Can you work these out from the model? Positions are in its coordinate system, mm. Round coordinates to 2 decimals unless told otherwise and drop trailing zeros. Loops run counter-clockwise (first coordinate to the right, second up) from the corner with the lowest first, then second, coordinate; pieces in that order, holes last. Notation, with made-up numbers: (-29, 72) -> (-7, 72) arc R21 ccw to (-7, 84) -> close; hole circle Ø9 at (-8.5, 80). An arc over 180 degrees is marked (long way). Answer as a JSON object with one key per item and string values.
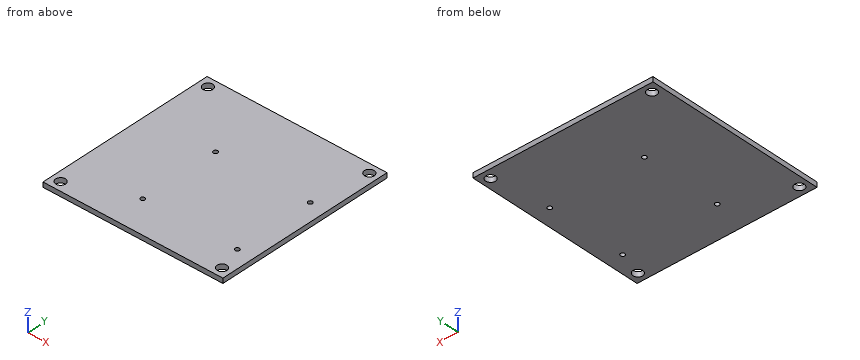
```python
from build123d import *

# Parameters (mm, degrees)
CROQUIS1_W              = 110.308657865
CROQUIS1_H              = 110.308657865
CROQUIS1_R              = 3
SALIENTE_EXTRUIR1_DEPTH = 3
CROQUIS3_R              = 1.35
CORTAR_EXTRUIR1_DEPTH   = 4


with BuildPart() as part:
    # Croquis1 → Saliente-Extruir1 (new body)
    with BuildSketch(Plane.XY.offset(1001.5)):
        with Locations((-24.891577249, 6.700344828)):
            Rectangle(CROQUIS1_W, CROQUIS1_H)
        with Locations((-74.389051931, 56.197819511)):
            Circle(CROQUIS1_R, mode=Mode.SUBTRACT)
        with Locations((24.605897435, -42.797129855)):
            Circle(CROQUIS1_R, mode=Mode.SUBTRACT)
        with Locations((-74.389051931, -42.797129855)):
            Circle(CROQUIS1_R, mode=Mode.SUBTRACT)
        with Locations((24.605897435, 56.197819511)):
            Circle(CROQUIS1_R, mode=Mode.SUBTRACT)
    extrude(amount=-SALIENTE_EXTRUIR1_DEPTH)

    # Croquis3 → Cortar-Extruir1 (cut, through all)
    with BuildSketch(Plane(origin=(0, 0, 998.5), x_dir=(-1, 0, 0), z_dir=(0, 0, -1))):
        with Locations((37.910718234, 21.399287334)):
            Circle(CROQUIS3_R)
        with Locations((37.910718234, -27.600712666)):
            Circle(CROQUIS3_R)
        with Locations((-20.089281766, -27.600712666)):
            Circle(CROQUIS3_R)
        with Locations((-20.089281766, 21.399287334)):
            Circle(CROQUIS3_R)
    extrude(amount=-CORTAR_EXTRUIR1_DEPTH, mode=Mode.SUBTRACT)


solid = part.part
```
Q1. If I drill on L1, parallel to Y at x = 20, z = 1001.35; L2, parallel to Y at x = -74, z = 1001.05, over which ranges is the centre line in solid material (lowest first)? Write a range as [from, to].
Determined:
{"L1": "[-48.45, -28.95], [-26.25, 20.05], [22.75, 61.85]", "L2": "[-48.45, -45.77], [-39.82, 53.22], [59.17, 61.85]"}
Q2. I want a section at B-B, the plane x = 23. Write out the boundary of the cut face in (y, z).
Determined:
{"outline": "(-48.45, 998.5) -> (-45.33, 998.5) -> (-45.33, 1001.5) -> (-48.45, 1001.5) -> close; (-40.26, 998.5) -> (53.66, 998.5) -> (53.66, 1001.5) -> (-40.26, 1001.5) -> close; (58.73, 998.5) -> (61.85, 998.5) -> (61.85, 1001.5) -> (58.73, 1001.5) -> close"}
Q3. I'm going to push flat-ended pins straight in: pin 1 (2.5 mm diameter, centred on x = 20.09, y = 21.4, fed in from +Z); pin 2 (8 mm diameter, centred on x = 24.61, y = 56.2, fed in from +Z). Where does each tip first touch, or does it pass through?
Determined:
{"pin 1": "through", "pin 2": "z = 1001.5"}
Q4. I want a section at A-A, the plane y = 54.5. Write out the boundary of the cut face in (x, z).
Determined:
{"outline": "(-80.05, 998.5) -> (-76.86, 998.5) -> (-76.86, 1001.5) -> (-80.05, 1001.5) -> close; (-71.92, 998.5) -> (22.13, 998.5) -> (22.13, 1001.5) -> (-71.92, 1001.5) -> close; (27.08, 998.5) -> (30.26, 998.5) -> (30.26, 1001.5) -> (27.08, 1001.5) -> close"}
